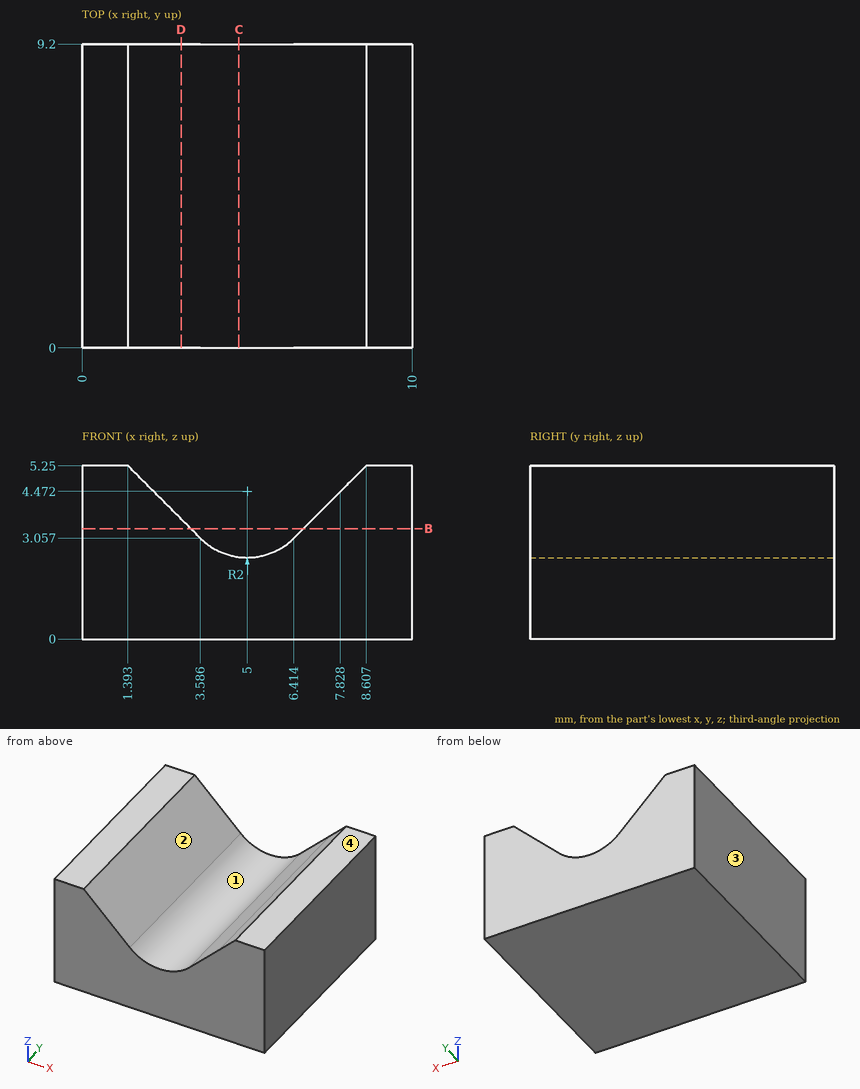
The drawing under review shows one solid part. Ordinate dimensions are in mm from its lowest x, y, z. Coordinates: 2 decimals unless noted, no trailing zeros. Order: outer loops, then holes, each group sorted by start corner. A loop starts at its lowest first (then second) coordinate and runs counter-clockwise, first axis right, second up. Notation, with made-up numbers: M 34,79 L 75,79 A20 ccw 75,85 Z; hole C -2,33.25 d2. An arc over 180 degrees is marked long. Use a Markdown table: item, result.
(1) Add section C-C (x = 4.75). Give the boundary of the cut face in (y, z), then the cut area to 3 significant figures.
Worked answers:
| item | result |
|---|---|
| outline | M 0,0 L 9.2,0 L 9.2,2.49 L 0,2.49 Z |
| area | 22.9 mm2 |
(2) Add section D-D (x = 3). Give the boundary of the cut face in (y, z).
Worked answers:
| item | result |
|---|---|
| outline | M 0,0 L 9.2,0 L 9.2,3.64 L 0,3.64 Z |
(3) Wall thickness on probe 1 along X at (y, z) = (1, 3.3) (1 decimal); probe 2 along X at (y, z) = (1, 2.7) (1 decimal); probe 3 along Z at (x, y) = (5, 1): over which ranges is each line inside the solid? List them lowest first.
Worked answers:
| item | result |
|---|---|
| probe 1 | x = 0 to 3.3, 6.7 to 10 |
| probe 2 | x = 0 to 4.1, 5.9 to 10 |
| probe 3 | z = 0 to 2.47 |
(4) Add section B-B (z = 3.35). Give the boundary of the cut face in (x, y).
Worked answers:
| item | result |
|---|---|
| outline | M 0,0 L 3.29,0 L 3.29,9.2 L 0,9.2 Z; M 6.71,0 L 10,0 L 10,9.2 L 6.71,9.2 Z |
(5) Draft analysis for pull direction X (two halves, no side actions). For the marked faces 1, 2, 3 and 4, state which applies: released by +X, released by -X, zero draft, split by the parting line, or undercut.
Worked answers:
| item | result |
|---|---|
| face 1 | undercut |
| face 2 | undercut |
| face 3 | released by -X |
| face 4 | zero draft |
